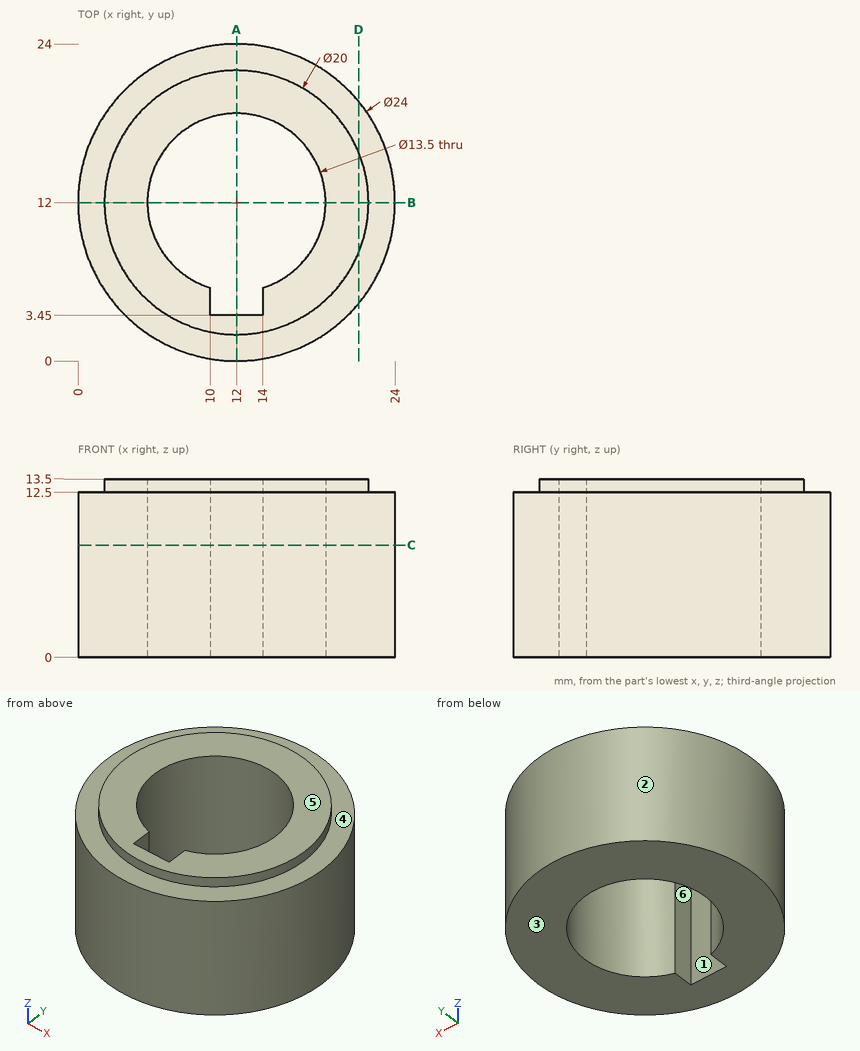
The drawing under review shows one solid part. Ordinate dimensions are in mm from its lowest x, y, z. A direction names the side the tool comes from. Coordinates: 2 decimals unless noted, no trailing zeros. Order: outer loops, then holes, each group sorted by start corner. A loop starts at its lowest first (then second) coordinate and runs counter-clockwise, first axis right, second up. Notation, with made-up numbers: M 41.5,54 L 56.5,54 A29 ccw 56.5,81 Z; hole C 10.5,-38 d4. An arc over 180 degrees is marked long. One line per question, with ' | ' between items.
(1) Add section B-B, the plane y = 12. Write out the cut boundary in (x, z).
Geometry results:
outline: M 0,0 L 5.25,0 L 5.25,13.5 L 2,13.5 L 2,12.5 L 0,12.5 Z; M 18.75,0 L 24,0 L 24,12.5 L 22,12.5 L 22,13.5 L 18.75,13.5 Z
(2) The part is to be moulded in two halves that separate along Y. For the marked faces 1, 2 and 3, say which applies: +Y half, -Y half, draft (parallel to the pull), parting line (faces both ways), or undercut.
Geometry results:
face 1: undercut | face 2: parting line | face 3: draft
(3) Insertion check: pin 1 (1.5 mm diameter, centred on y = 19.5, z = 2, fed in from +X); pin 2 (4 mm diameter, centred on x = 16.5, z = 8, fed in from -Y); pin 3 (4 mm diameter, centred on x = 6.5, z = 7.5, fed in from +Y). Each pin has a flat end and moves straight along its axis. Give the tip position at first contact, or say it passes through.
Geometry results:
pin 1: stops at x = 21.92 | pin 2: stops at y = 0.26 | pin 3: stops at y = 23.48
(4) Add section C-C, the plane z = 8.5. Write out the cut boundary in (x, y), then the cut area to 3 significant figures.
Geometry results:
outline: C 12,12 d24; hole M 10,3.45 L 14,3.45 L 14,5.55 A6.75 ccw long 10,5.55 Z | area: 302 mm²
(5) For probe 1 along Y at (x, z) = (12, 8.25); probe 2 along X at (y, z) = (12.25, 1.75); probe 3 along X at (y, z) = (10.25, 1.5), list the stretches that pass through material, from the lowest coordinate up. Write a range as from..to.
Geometry results:
probe 1: y = 0..3.45, 18.75..24 | probe 2: x = 0..5.25, 18.75..24 | probe 3: x = 0.13..5.48, 18.52..23.87
(6) Add section D-D, the plane x = 21.25. Write out the cut boundary in (y, z).
Geometry results:
outline: M 4.36,0 L 19.64,0 L 19.64,12.5 L 15.8,12.5 L 15.8,13.5 L 8.2,13.5 L 8.2,12.5 L 4.36,12.5 Z
(7) Add section A-A, the plane x = 12. Write out the cut boundary in (y, z), then the cut area to 3 significant figures.
Geometry results:
outline: M 0,0 L 3.45,0 L 3.45,13.5 L 2,13.5 L 2,12.5 L 0,12.5 Z; M 18.75,0 L 24,0 L 24,12.5 L 22,12.5 L 22,13.5 L 18.75,13.5 Z | area: 113 mm²
(8) Machinability: for the marked faces 4, 5 and 6, which of the approach directions +Z, -Z, +X, -X, +Y, -Y give a long, thin tool a straight path to every point of the face, cutting with its end or side? Answer none if there is none.
Geometry results:
face 4: +Z | face 5: +Z, +X, -X, +Y, -Y | face 6: +Z, -Z
